The model under review builds one solid part; all positions refer to its coordinate system, in mm. A direction names the side the tool comes from. Round coordinates to 2 decimals unless told otherwise and drop trailing zeros. Order: outer loops, then holes, each group sorted by start corner. A loop starts at its lowest first (then second) coordinate and runs counter-clockwise, first axis right, second up. Notation, with made-up numbers: M 71,-27 L 97,-27 A21 cw 97,-11 Z; hole C 74,-26 d3. An arc over 180 degrees is marked long. Use a Markdown table: item, result. Add a question column.
1. Consider section B-B on z = 0. State the section outline as (x, y) points, then the cut area to 3 significant figures.
2. Consider section C-C on y = -17.75. State the section outline as (x, z) points.
3. For faces 1 (the cylindrical face through (-3, -10, 0)), 2 (the flat face through (-11.5, -10, 5.9)), list the 3-axis set-ups (+Z, -Z, +X, -X, +Y, -Y) from which the entire face can be reached by the end or side of a thin tool; tool diameter is ignored.
4. To check wall thickness, follow probe 1 along Z at (x, y) = (0, -12.5); probe 2 along Y at (x, z) = (-22, -11.5); probe 3 along Z at (x, y) = (2.5, -5.25). State the ranges of each line that lie inside material, in increasing order.
5. Consider section A-A on x = 0. State the section outline as (y, z) points.
6. Consider section D-D on x = -10. State the section outline as (y, z) points, then the cut area to 3 significant figures.
7. Insertion check: P1, Ø4, axis at x = -2, y = -16.5, coming from the +Z side; P2, Ø1.5, axis at x = 14.5, z = 15.5, coming from the -Y side; P3, Ø2, axis at x = -10.5, y = -14, coming from the -Z side. Each pin has a flat end and moves straight along its axis. Give the tip position at first contact, or say it passes through.
from build123d import *

# Parameters (mm, degrees)
SKETCH_R     = 25
PAD_DEPTH    = 10
SKETCH001_R  = 12.5
PAD001_DEPTH = 10
SKETCH002_R  = 3
POCKET_DEPTH = 20


with BuildPart() as part:
    # Sketch → Pad (new body)
    with BuildSketch(Plane.XZ):
        Circle(SKETCH_R)
    extrude(amount=PAD_DEPTH)

    # Sketch001 (on Face3 of Pad) → Pad001 (join)
    with BuildSketch(Plane.XZ.offset(10)):
        Circle(SKETCH001_R)
    extrude(amount=PAD001_DEPTH)

    # Sketch002 (on Face5 of Pad001) → Pocket (cut)
    with BuildSketch(Plane.XZ.offset(20)):
        Circle(SKETCH002_R)
    extrude(amount=-POCKET_DEPTH, mode=Mode.SUBTRACT)


solid = part.part
Answer block:
| question | item | result |
|---|---|---|
| 1 | outline | M -25,-10 L -12.5,-10 L -12.5,-20 L -3,-20 L -3,0 L -25,0 Z; M 3,-20 L 12.5,-20 L 12.5,-10 L 25,-10 L 25,0 L 3,0 Z |
| 1 | area | 630 mm^2 |
| 2 | outline | C 0,0 d25; hole C 0,0 d6 |
| 3 | face 1 | +Y, -Y |
| 3 | face 2 | -Y |
| 4 | probe 1 | -12.5 to -3, 3 to 12.5 |
| 4 | probe 2 | -10 to 0 |
| 4 | probe 3 | -24.87 to -1.66, 1.66 to 24.87 |
| 5 | outline | M -20,-12.5 L -10,-12.5 L -10,-25 L 0,-25 L 0,-3 L -20,-3 Z; M -20,3 L 0,3 L 0,25 L -10,25 L -10,12.5 L -20,12.5 Z |
| 6 | outline | M -20,-7.5 L -10,-7.5 L -10,-22.91 L 0,-22.91 L 0,22.91 L -10,22.91 L -10,7.5 L -20,7.5 Z |
| 6 | area | 608 mm^2 |
| 7 | P1 | z = 12.5 |
| 7 | P2 | y = -10 |
| 7 | P3 | z = -8.12 |
